Read the model definition and answer for the solid it produces. Units are mm, in the model's axes. A direction names the side the tool comes from. Give positions to 0.01 mm unless a question says otherwise; leave off trailing zeros. Loops run counter-clockwise (first coordinate to the right, second up) from the corner with the lowest first, then second, coordinate; pieces in that order, holes last. Notation, with made-up numbers: M 13.25,12 L 46.25,12 A8 ccw 46.25,22 Z; hole C 77.5,2 d5. An arc over 180 degrees is marked long. Return JSON: item names as keys, results as strings. Group by question number.
```python
from build123d import *

# Parameters (mm, degrees)
SKETCH1_W           = 65
SKETCH1_H           = 95.5
BOSS_EXTRUDE1_DEPTH = 2
SKETCH1_3_W         = 62.5
SKETCH1_3_H         = 92.5
BOSS_EXTRUDE2_DEPTH = 6
BOSS_EXTRUDE3_START = 6
SKETCH2_4_W         = 19.3
SKETCH2_4_H         = 19.3
BOSS_EXTRUDE3_DEPTH = 8
SKETCH2_R           = 7.65
CUT_EXTRUDE1_DEPTH  = 19.5
CUT_EXTRUDE2_START  = 40
CUT_EXTRUDE2_DEPTH  = 39
CUT_EXTRUDE3_DEPTH  = 10
FILLET1_R           = 4
SKETCH5_W           = 19.3
SKETCH5_H           = 19.3
CUT_EXTRUDE5_DEPTH  = 4
FILLET2_R           = 2


with BuildPart() as part:
    # Sketch1 → Boss-Extrude1 (new body)
    with BuildSketch(Plane(origin=(0, 0, 0), x_dir=(1, 0, 0), z_dir=(0, 1, 0))):
        Rectangle(SKETCH1_W, SKETCH1_H)
    extrude(amount=BOSS_EXTRUDE1_DEPTH)

    # Sketch1<3> → Boss-Extrude2 (add)
    with BuildSketch(Plane(origin=(0, 0, 0), x_dir=(1, 0, 0), z_dir=(0, 1, 0))):
        Rectangle(SKETCH1_3_W, SKETCH1_3_H)
    extrude(amount=BOSS_EXTRUDE2_DEPTH)

    # Sketch2<4> → Boss-Extrude3 (add)
    with BuildSketch(Plane(origin=(0, 0, 0), x_dir=(1, 0, 0), z_dir=(0, 1, 0)).offset(BOSS_EXTRUDE3_START)):
        Rectangle(SKETCH2_4_W, SKETCH2_4_H)
    extrude(amount=BOSS_EXTRUDE3_DEPTH)

    # Sketch2 → Cut-Extrude1 (cut, symmetric)
    with BuildSketch(Plane(origin=(0, 0, 0), x_dir=(1, 0, 0), z_dir=(0, 1, 0))):
        with Locations(Location((0, 0, 0), (0, 0, 270))):
            Circle(SKETCH2_R)
    extrude(amount=CUT_EXTRUDE1_DEPTH, both=True, mode=Mode.SUBTRACT)

    # Sketch2<3> → Cut-Extrude2 (cut)
    with BuildSketch(Plane(origin=(0, 0, 0), x_dir=(1, 0, 0), z_dir=(0, 1, 0)).offset(CUT_EXTRUDE2_START)):
        with BuildLine():
            Line((9e-09, 7.65), (-7.65, 7.65))
            Line((-7.65, 7.65), (-7.65, 0))
            ThreePointArc((-7.65, 0), (-5.409366873, 5.409366879), (9e-09, 7.65))
        make_face()
        with BuildLine():
            Line((7.65, 7.65), (9e-09, 7.65))
            ThreePointArc((9e-09, 7.65), (7.65, 0), (9e-09, -7.65))
            Line((9e-09, -7.65), (7.65, -7.65))
            Line((7.65, -7.65), (7.65, -0.65))
            ThreePointArc((7.65, -0.65), (8.519734544, 1), (7.65, 2.65))
            Line((7.65, 2.65), (7.65, 7.65))
        make_face()
        with BuildLine():
            ThreePointArc((9e-09, -7.65), (-5.409366873, -5.409366879), (-7.65, 0))
            Line((-7.65, 0), (-7.65, -7.65))
            Line((-7.65, -7.65), (9e-09, -7.65))
        make_face()
    extrude(amount=-CUT_EXTRUDE2_DEPTH, mode=Mode.SUBTRACT)

    # Sketch3 → Cut-Extrude3 (cut)
    with BuildSketch(Plane(origin=(0, 0, 0), x_dir=(1, 0, 0), z_dir=(0, 1, 0))):
        with BuildLine():
            Line((-30.433287704, 49.156662819), (-34.566712296, 46.343337181))
            Line((-34.566712296, 46.343337181), (-30.346723838, 40.143200294))
            ThreePointArc((-30.346723838, 40.143200294), (-26.873348724, 39.483150817), (-26.213299247, 42.956525932))
            Line((-26.213299247, 42.956525932), (-30.433287704, 49.156662819))
        make_face()
        with BuildLine():
            Line((34.566712296, 46.343337181), (30.433287704, 49.156662819))
            Line((30.433287704, 49.156662819), (26.213299247, 42.956525932))
            ThreePointArc((26.213299247, 42.956525932), (26.873348724, 39.483150817), (30.346723838, 40.143200294))
            Line((30.346723838, 40.143200294), (34.566712296, 46.343337181))
        make_face()
        with BuildLine():
            Line((-30.346723838, -40.143200294), (-34.566712296, -46.343337181))
            Line((-34.566712296, -46.343337181), (-30.433287704, -49.156662819))
            Line((-30.433287704, -49.156662819), (-26.213299247, -42.956525932))
            ThreePointArc((-26.213299247, -42.956525932), (-26.873348724, -39.483150817), (-30.346723838, -40.143200294))
        make_face()
        with BuildLine():
            Line((26.213299247, -42.956525932), (30.433287704, -49.156662819))
            Line((30.433287704, -49.156662819), (34.566712296, -46.343337181))
            Line((34.566712296, -46.343337181), (30.346723838, -40.143200294))
            ThreePointArc((30.346723838, -40.143200294), (26.873348724, -39.483150817), (26.213299247, -42.956525932))
        make_face()
    extrude(amount=CUT_EXTRUDE3_DEPTH, mode=Mode.SUBTRACT)

    # Fillet1
    # the kernel refuses this fillet: 4 mm, written as the material it takes off along each edge
    with BuildSketch(Plane(origin=(-36.876651276, 6, 49.737170606), x_dir=(0, -1, 0), z_dir=(0.5626651276372232, 0, -0.826684918297768)), Plane(origin=(30.346723838, 6, 40.143200294), x_dir=(0, -1, 0), z_dir=(0.5626651276372238, 0, 0.8266849182977677)), Plane(origin=(36.876651276, 6, -49.737170606), x_dir=(0, -1, 0), z_dir=(-0.562665127637224, 0, 0.8266849182977676)), Plane(origin=(-30.346723838, 6, -40.143200294), x_dir=(0, -1, 0), z_dir=(-0.5626651276372242, 0, -0.8266849182977674))) as fillet1_piece_1:
        with BuildLine():
            CenterArc((FILLET1_R, FILLET1_R), FILLET1_R, 180, 90)
            Line((0, FILLET1_R), (0, 0))
            Line((0, 0), (FILLET1_R, 0))
        make_face()
    extrude(amount=11.605353019, mode=Mode.SUBTRACT)
    with BuildSketch(Plane(origin=(-26.213299247, 6, 42.956525932), x_dir=(0, -1, 0), z_dir=(-0.5626651276372243, 0, 0.8266849182977672)), Plane(origin=(34.081582088, 6, 54.516849183), x_dir=(0, -1, 0), z_dir=(-0.5626651276372246, 0, -0.826684918297767)), Plane(origin=(26.213299247, 6, -42.956525932), x_dir=(0, -1, 0), z_dir=(0.5626651276372232, 0, -0.826684918297768)), Plane(origin=(-34.081582088, 6, -54.516849183), x_dir=(0, -1, 0), z_dir=(0.562665127637224, 0, 0.8266849182977676))) as fillet1_piece_2:
        with BuildLine():
            CenterArc((FILLET1_R, FILLET1_R), FILLET1_R, 180, 90)
            Line((0, FILLET1_R), (0, 0))
            Line((0, 0), (FILLET1_R, 0))
        make_face()
    extrude(amount=13.983953251, mode=Mode.SUBTRACT)
    with BuildSketch(Plane(origin=(-28.280011543, 6, 41.549863113), x_dir=(-0.8266849182977704, 0, -0.5626651276372198), z_dir=(-0.5626651276372198, 0, 0.8266849182977704))) as fillet1_piece_3:
        with BuildLine():
            CenterArc((2.5 + FILLET1_R, FILLET1_R), FILLET1_R, 180, 90)
            Line((2.5 + FILLET1_R, 0), (2.5, 0))
            Line((2.5, 0), (2.5, FILLET1_R))
        make_face()
    revolve(axis=Axis((-28.280011543, 6, 41.549863113), (0, -1, 0)), revolution_arc=180, mode=Mode.SUBTRACT)
    with BuildSketch(Plane(origin=(28.280011543, 6, 41.549863113), x_dir=(-0.8266849182977659, 0, 0.5626651276372262), z_dir=(0.5626651276372262, 0, 0.8266849182977659))) as fillet1_piece_4:
        with BuildLine():
            CenterArc((2.5 + FILLET1_R, FILLET1_R), FILLET1_R, 180, 90)
            Line((2.5 + FILLET1_R, 0), (2.5, 0))
            Line((2.5, 0), (2.5, FILLET1_R))
        make_face()
    revolve(axis=Axis((28.280011543, 6, 41.549863113), (0, -1, 0)), revolution_arc=180, mode=Mode.SUBTRACT)
    with BuildSketch(Plane(origin=(28.280011543, 6, -41.549863113), x_dir=(0.826684918297769, 0, 0.5626651276372218), z_dir=(0.5626651276372218, 0, -0.826684918297769))) as fillet1_piece_5:
        with BuildLine():
            CenterArc((2.5 + FILLET1_R, FILLET1_R), FILLET1_R, 180, 90)
            Line((2.5 + FILLET1_R, 0), (2.5, 0))
            Line((2.5, 0), (2.5, FILLET1_R))
        make_face()
    revolve(axis=Axis((28.280011543, 6, -41.549863113), (0, -1, 0)), revolution_arc=180, mode=Mode.SUBTRACT)
    with BuildSketch(Plane(origin=(-28.280011543, 6, -41.549863113), x_dir=(0.8266849182977655, 0, -0.562665127637227), z_dir=(-0.562665127637227, 0, -0.8266849182977655))) as fillet1_piece_6:
        with BuildLine():
            CenterArc((2.5 + FILLET1_R, FILLET1_R), FILLET1_R, 180, 90)
            Line((2.5 + FILLET1_R, 0), (2.5, 0))
            Line((2.5, 0), (2.5, FILLET1_R))
        make_face()
    revolve(axis=Axis((-28.280011543, 6, -41.549863113), (0, -1, 0)), revolution_arc=180, mode=Mode.SUBTRACT)

    # Sketch5 → Cut-Extrude5 (cut)
    with BuildSketch(Plane(origin=(0, 6, 0), x_dir=(1, 0, 0), z_dir=(0, 1, 0))):
        with BuildLine():
            Line((-20.220280729, -44.25), (20.220280729, -44.25))
            ThreePointArc((20.220280729, -44.25), (21.675717981, -36.198853249), (29.25, -33.105390223))
            Line((29.25, -33.105390223), (29.25, 33.105390223))
            ThreePointArc((29.25, 33.105390223), (21.675717981, 36.198853249), (20.220280729, 44.25))
            Line((20.220280729, 44.25), (-20.220280729, 44.25))
            ThreePointArc((-20.220280729, 44.25), (-21.675717981, 36.198853249), (-29.25, 33.105390223))
            Line((-29.25, 33.105390223), (-29.25, -33.105390223))
            ThreePointArc((-29.25, -33.105390223), (-21.675717981, -36.198853249), (-20.220280729, -44.25))
        make_face()
        Rectangle(SKETCH5_W, SKETCH5_H, mode=Mode.SUBTRACT)
    extrude(amount=-CUT_EXTRUDE5_DEPTH, mode=Mode.SUBTRACT)

    # Fillet2
    fillet2_edges = [part.edges().sort_by_distance(p)[0] for p in [
        (0, 2, -9.65),
        (-9.65, 2, 0),
        (0, 2, 9.65),
        (9.65, 2, 0),
    ]]
    fillet(fillet2_edges, radius=FILLET2_R)


solid = part.part
```
1. The mould has two halves that part along X. Classify faces 6 (the cylindrical face through (0.16, 2.57, 10.25)), 7 (the flat face through (0, 14, 8)), 8 (the cylindrical face through (26.45, 4.33, -44.636)): +X half, -X half, draft (parallel to the pull), parting line (faces both ways), or undercut.
2. Find section A-A (x = -3.5). Write down the section's boundary in (y, z), and give its area (3 significant figures).
3. Flat-ended cylindrical pins translate along their axes: P1, Ø1, axis at x = -15, z = -27, coming from the +Y side; P2, Ø1.2, axis at y = 3.5, z = 1, coming from the +X side; P3, Ø4.5, axis at x = 11, y = 5, coming from the +Z side. Find the tip coordinate at first contact, or state that the pin passes through.
4. Find section B-B (y = 12.75). Write down the section's boundary in (x, z).
5. For faces 1 (the flat face through (0, 4, 46.25)), 2 (the cylindrical face through (30.84, 3.18, 40.55)), 3 (the flat face through (31.25, 4, 1)), 4 (the cylindrical face through (-26.45, 4.33, 44.636)), 5 (the flat face through (-6, 1, -6)), determine the directions among +Z, -Z, +X, -X, +Y, -Y from which every point of the face is accessible in a straight line to the end or side of a thin tool.
6. Find section C-C (x = 16). Write down the section's boundary in (y, z), and give its area (3 significant figures).
7. Straight lines are drawn through the part: line 1 along X through (y, z) = (5.75, 5.5); line 2 along X through (y, z) = (0.4, 0); line 3 along X through (y, z) = (4.25, -16). For each, find the intervals that lie inside material, in ascending order.
Result:
{
 "1": {"face 6": "undercut", "face 7": "draft", "face 8": "+X half"},
 "2": {"outline": "M 0,-47.75 L 2,-47.75 L 2,-46.25 L 6,-46.25 L 6,-44.25 L 2,-44.25 L 2,-11.65 A2 cw 4,-9.65 L 14,-9.65 L 14,-7.65 L 1,-7.65 L 1,-6.8 L 0,-6.8 Z; M 0,6.8 L 1,6.8 L 1,7.65 L 14,7.65 L 14,9.65 L 4,9.65 A2 cw 2,11.65 L 2,44.25 L 6,44.25 L 6,46.25 L 2,46.25 L 2,47.75 L 0,47.75 Z", "area": "228 mm2"},
 "3": {"P1": "stops at y = 2", "P2": "stops at x = 31.25", "P3": "stops at z = 46.25"},
 "4": {"outline": "M -9.65,-9.65 L 9.65,-9.65 L 9.65,9.65 L -9.65,9.65 Z; hole M -7.65,-7.65 L 7.65,-7.65 L 7.65,-2.65 A2 ccw 7.65,0.65 L 7.65,7.65 L -7.65,7.65 Z"},
 "5": {"face 1": "+Z, +X, -X, +Y", "face 2": "+Z, +Y", "face 3": "+Z, -Z, +X, +Y", "face 4": "-X, +Y", "face 5": "+Y"},
 "6": {"outline": "M 0,-47.75 L 2,-47.75 L 2,-46.25 L 6,-46.25 L 6,-44.25 L 2,-44.25 L 2,44.25 L 6,44.25 L 6,46.25 L 2,46.25 L 2,47.75 L 0,47.75 Z", "area": "207 mm2"},
 "7": {"line 1": "x = -31.25 to -29.25, -9.65 to -7.65, 7.65 to 9.65, 29.25 to 31.25", "line 2": "x = -32.5 to -7.65, 7.65 to 32.5", "line 3": "x = -31.25 to -29.25, 29.25 to 31.25"}
}
